Autodesk Inventor part; units mm, degrees
ref_plane "YZ Plane" through (0, 0, 0) normal (1, 0, 0) x (0, 1, 0)
ref_plane "XZ Plane" through (0, 0, 0) normal (0, 1, 0) x (-1, 0, 0)
ref_plane "XY Plane" through (0, 0, 0) normal (0, 0, 1) x (1, 0, 0)
sketch "Sketch1" plane through (0, 0, 0) normal (0, 1, 0) x (-1, 0, 0)
  line L0 (4.85, 6.35) -> (-4.85, 6.35)
  line L1 (-6.35, 4.85) -> (-6.35, -4.85)
  line L2 (-4.85, -6.35) -> (4.85, -6.35)
  line L3 (6.35, -4.85) -> (6.35, 4.85)
  line L4 (6.35, 6.35) -> (-6.35, -6.35) construction
  line L5 (-6.35, 6.35) -> (6.35, -6.35) construction
  line L6 (6.35, -4.85) -> (4.85, -6.35)
  line L7 (-4.85, -6.35) -> (-6.35, -4.85)
  line L8 (-4.85, 6.35) -> (-6.35, 4.85)
  line L9 (6.35, 4.85) -> (4.85, 6.35)
  line L10 (4.32, 4.32) -> (-4.32, 4.32) construction
  line L11 (-4.32, 4.32) -> (-4.32, -4.32) construction
  line L12 (-4.32, -4.32) -> (4.32, -4.32) construction
  line L13 (4.32, -4.32) -> (4.32, 4.32) construction
  line L14 (4.32, 4.32) -> (-4.32, -4.32) construction
  line L15 (-4.32, 4.32) -> (4.32, -4.32) construction
  circle A0 centre (0, 0) radius 1.3272
  dimension "d0" = 12.7
  dimension "d1" = 12.7
  dimension "d5" = 9.7
  dimension "d6" = 1.5
  dimension "d7" = 8.64
  dimension "d8" = 8.64
  dimension "d9" = 2.6543
extrude "Extrusion1" add sketch "Sketch1" along normal blind 1.65
sketch "Sketch2" plane through (0, 1.65, 0) normal (0, 1, 0) x (1, 0, 0)
  circle A0 centre (0, 0) radius 1.3272
  line L0 (-4.32, -4.32) -> (4.32, -4.32) construction
  line L1 (4.32, -4.32) -> (4.32, 4.32) construction
  line L2 (4.32, 4.32) -> (-4.32, 4.32) construction
  line L3 (-4.32, 4.32) -> (-4.32, -4.32) construction
  line L4 (-4.32, -4.32) -> (4.32, 4.32) construction
  line L5 (4.32, -4.32) -> (-4.32, 4.32) construction
  dimension "d12" = 8.64
  dimension "d13" = 8.64
hole "Hole1" at (-4.32, 1.65, -4.32) at (4.32, 1.65, -4.32) at (4.32, 1.65, 4.32) at (-4.32, 1.65, 4.32) direction (0, -1, 0) diameter 2.64 depth 1.65 tip angle 118
sketch "Sketch3" plane through (0, 1.65, 0) normal (0, 1, 0) x (1, 0, 0)
  circle A0 centre (0, 0) radius 1.3272
  circle A1 centre (0, 0) radius 3.145
  dimension "d21" = 6.29
extrude "Extrusion2" add sketch "Sketch3" along normal blind 7.93 contours A0 | A1
thread "Thread1"
chamfer "Chamfer1" distance 0.3 angle 45 1 edges at (-3.145, 9.58, 0)
sketch "Sketch4" plane through (0, 9.58, 0) normal (0, 1, 0) x (1, 0, 0)
  circle A0 centre (0, 0) radius 2.845
  circle A1 centre (0, 0) radius 2.75
  dimension "d30" = 5.5
extrude "Extrusion3" cut sketch "Sketch4" against normal blind 3 contours A1
sketch "Sketch5" plane through (0, 1.65, 0) normal (0, -1, 0) x (1, 0, 0)
  circle A0 centre (0, 0) radius 1.3272
  circle A1 centre (0, 0) radius 0.254
  dimension "d33" = 0.508
extrude "Extrusion4" cut sketch "Sketch5" against normal blind 6 contours A1
sketch "Sketch6" plane through (0, 6.58, 0) normal (0, 1, 0) x (1, 0, 0)
  circle A0 centre (0, 0) radius 0.254
  circle A1 centre (0, 0) radius 2.75
  circle A2 centre (0, 0) radius 0.5
  dimension "d36" = 1
extrude "Extrusion5" cut sketch "Sketch6" against normal blind 2 contours A2
sketch "Sketch7" plane through (0, 0, 0) normal (0, -1, 0) x (1, 0, 0)
  line L0 (-6.35, -6.35) -> (6.35, -6.35)
  line L1 (6.35, -6.35) -> (6.35, 6.35)
  line L2 (6.35, 6.35) -> (-6.35, 6.35)
  line L3 (-6.35, 6.35) -> (-6.35, -6.35)
  circle A0 centre (0, 0) radius 0.254
  line L4 (-6.35, -6.35) -> (6.35, 6.35) construction
  line L5 (6.35, -6.35) -> (-6.35, 6.35) construction
extrude "Extrusion6" cut sketch "Sketch7" against normal blind 2
properties part number "sma"
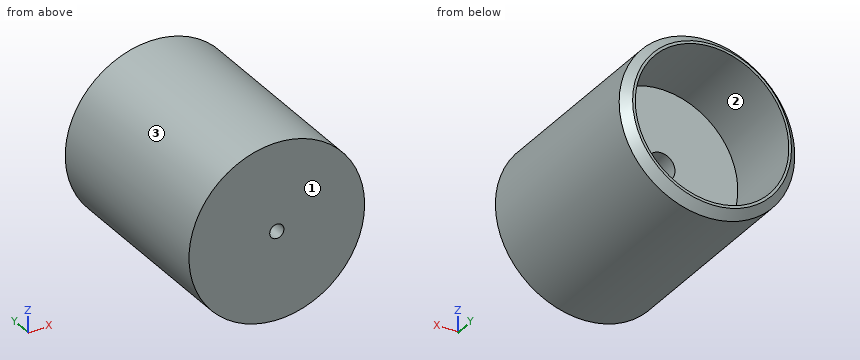
Verification items for the finished model (mm, model axes). Face numbers are marked on the shaded views. Give positions to 0.01 mm unless a question says otherwise; leave off trailing zeros. Write each loop counter-clockwise with the first axis right and the second up, starting at its lowest first coordinate (ties: lowest second). Pieces come first, ordered by that corner, then holes. Notation, with made-up numbers: (65.25, 73.25) - (107.25, 73.25) arc R22 cw to (107.25, 91.25) - close; hole circle Ø7 at (-12, 61.25). An arc over 180 degrees is marked (long way). Put each result on its own line as item: value.
Q1. Section check D-D on y = 2.5. Record the cut outline in (x, z) (3 decimals).
Result:
outline: circle Ø6.29 at (0, 0); hole circle Ø0.508 at (0, 0)
Q2. Section check A-A on z = 0. Record the cut outline in (x, y) (3 decimals).
Result:
outline: (-3.145, 2) - (-0.254, 2) - (-0.254, 4.58) - (-0.5, 4.58) - (-0.5, 6.58) - (-2.75, 6.58) - (-2.75, 9.58) - (-2.845, 9.58) - (-3.145, 9.28) - close; (0.254, 2) - (3.145, 2) - (3.145, 9.28) - (2.845, 9.58) - (2.75, 9.58) - (2.75, 6.58) - (0.5, 6.58) - (0.5, 4.58) - (0.254, 4.58) - close
Q3. Section check B-B on x = 0. Record the cut outline in (y, z) (3 decimals), and give its area (3 significant figures).
Result:
outline: (2, -3.145) - (9.28, -3.145) - (9.58, -2.845) - (9.58, -2.75) - (6.58, -2.75) - (6.58, -0.5) - (4.58, -0.5) - (4.58, -0.254) - (2, -0.254) - close; (2, 0.254) - (4.58, 0.254) - (4.58, 0.5) - (6.58, 0.5) - (6.58, 2.75) - (9.58, 2.75) - (9.58, 2.845) - (9.28, 3.145) - (2, 3.145) - close
area: 27.8 mm2
Q4. Depth check by flat-ended pin: P1, Ø1, axis at y = 4, z = -1, coming from the +X side (3 decimals); P2, Ø3, axis at x = -2, y = 5, coming from the -Z side (3 decimals); P3, Ø2, axis at x = -2, y = 6, coming from the +Z side. Enter the tip coordinate at first touch or a pass-through.
Result:
P1: x = 3.105
P2: z = -3.105
P3: z = 2.98
Q5. Section check C-C on y = 7.25. Record the cut outline in (x, z) (3 decimals).
Result:
outline: circle Ø6.29 at (0, 0); hole circle Ø5.5 at (0, 0)
Q6. Mould release check, pull along Z, two halves, no side actions. Record for the marked faces 1, 2 and 3: released by +Z, released by -Z, zero draft, split by the parting line, or undercut.
Result:
face 1: zero draft
face 2: undercut
face 3: split by the parting line
Q7. Scan lines: probe 1 along Z at (x, y) = (0, 4.5) (3 decimals); probe 2 along Z at (x, y) = (0, 7.3) (3 decimals). Record each from-to range of solid material in increasing order. Write a range as from..to.
Result:
probe 1: -3.145..-0.254, 0.254..3.145
probe 2: -3.145..-2.75, 2.75..3.145
